```python
from build123d import *

# Parameters (mm, degrees)
SKETCH1_W           = 203.2
SKETCH1_H           = 60.2
BOSS_EXTRUDE1_DEPTH = 3
SKETCH5_R           = 2.5
CUT_EXTRUDE1_DEPTH  = 3
SKETCH7_R           = 2.5
CUT_EXTRUDE2_DEPTH  = 3
CUT_EXTRUDE3_DEPTH  = 3


with BuildPart() as part:
    # Sketch1 → Boss-Extrude1 (new body)
    with BuildSketch(Plane(origin=(0, 0, 0), x_dir=(1, 0, 0), z_dir=(0, 1, 0))):
        Rectangle(SKETCH1_W, SKETCH1_H)
    extrude(amount=BOSS_EXTRUDE1_DEPTH)

    # Sketch5 → Cut-Extrude1 (cut)
    with BuildSketch(Plane(origin=(0, 3, 0), x_dir=(1, 0, 0), z_dir=(0, 1, 0))):
        with Locations(Location((74.1, 3.6, 0), (0, 0, 270))):
            Circle(SKETCH5_R)
    extrude(amount=-CUT_EXTRUDE1_DEPTH, mode=Mode.SUBTRACT)

    # Sketch7 → Cut-Extrude2 (cut)
    with BuildSketch(Plane(origin=(0, 3, 0), x_dir=(1, 0, 0), z_dir=(0, 1, 0))):
        with Locations(Location((74.1, -7.1, 0), (0, 0, 270))):
            Circle(SKETCH7_R)
    extrude(amount=-CUT_EXTRUDE2_DEPTH, mode=Mode.SUBTRACT)

    # Sketch8 → Cut-Extrude3 (cut)
    with BuildSketch(Plane(origin=(0, 3, 0), x_dir=(1, 0, 0), z_dir=(0, 1, 0))):
        with BuildLine():
            Line((46.873111379, 15.864980996), (61.83445164, 0.932505799))
            ThreePointArc((61.83445164, 0.932505799), (61.836499957, -1.188813555), (59.715180603, -1.190861873))
            Line((59.715180603, -1.190861873), (44.753840342, 13.741613324))
            ThreePointArc((44.753840342, 13.741613324), (44.751792025, 15.862932678), (46.873111379, 15.864980996))
        make_face()
        with BuildLine():
            Line((36.873111379, 15.864980996), (51.83445164, 0.932505799))
            ThreePointArc((51.83445164, 0.932505799), (51.836499957, -1.188813555), (49.715180603, -1.190861873))
            Line((49.715180603, -1.190861873), (34.753840342, 13.741613324))
            ThreePointArc((34.753840342, 13.741613324), (34.751792025, 15.862932678), (36.873111379, 15.864980996))
        make_face()
        with BuildLine():
            Line((26.873111379, 15.864980996), (41.83445164, 0.932505799))
            ThreePointArc((41.83445164, 0.932505799), (41.836499957, -1.188813555), (39.715180603, -1.190861873))
            Line((39.715180603, -1.190861873), (24.753840342, 13.741613324))
            ThreePointArc((24.753840342, 13.741613324), (24.751792025, 15.862932678), (26.873111379, 15.864980996))
        make_face()
        with BuildLine():
            Line((16.873111379, 15.864980996), (31.83445164, 0.932505799))
            ThreePointArc((31.83445164, 0.932505799), (31.836499957, -1.188813555), (29.715180603, -1.190861873))
            Line((29.715180603, -1.190861873), (14.753840342, 13.741613324))
            ThreePointArc((14.753840342, 13.741613324), (14.751792025, 15.862932678), (16.873111379, 15.864980996))
        make_face()
        with BuildLine():
            Line((36.873111379, -4.135019004), (51.83445164, -19.067494201))
            ThreePointArc((51.83445164, -19.067494201), (51.836499957, -21.188813555), (49.715180603, -21.190861873))
            Line((49.715180603, -21.190861873), (34.753840342, -6.258386676))
            ThreePointArc((34.753840342, -6.258386676), (34.751792025, -4.137067322), (36.873111379, -4.135019004))
        make_face()
        with BuildLine():
            Line((26.873111379, -4.135019004), (41.83445164, -19.067494201))
            ThreePointArc((41.83445164, -19.067494201), (41.836499957, -21.188813555), (39.715180603, -21.190861873))
            Line((39.715180603, -21.190861873), (24.753840342, -6.258386676))
            ThreePointArc((24.753840342, -6.258386676), (24.751792025, -4.137067322), (26.873111379, -4.135019004))
        make_face()
        with BuildLine():
            Line((16.873111379, -4.135019004), (31.83445164, -19.067494201))
            ThreePointArc((31.83445164, -19.067494201), (31.836499957, -21.188813555), (29.715180603, -21.190861873))
            Line((29.715180603, -21.190861873), (14.753840342, -6.258386676))
            ThreePointArc((14.753840342, -6.258386676), (14.751792025, -4.137067322), (16.873111379, -4.135019004))
        make_face()
        with BuildLine():
            Line((46.873111379, -4.135019004), (61.83445164, -19.067494201))
            ThreePointArc((61.83445164, -19.067494201), (61.836499957, -21.188813555), (59.715180603, -21.190861873))
            Line((59.715180603, -21.190861873), (44.753840342, -6.258386676))
            ThreePointArc((44.753840342, -6.258386676), (44.751792025, -4.137067322), (46.873111379, -4.135019004))
        make_face()
    extrude(amount=-CUT_EXTRUDE3_DEPTH, mode=Mode.SUBTRACT)


solid = part.part
```
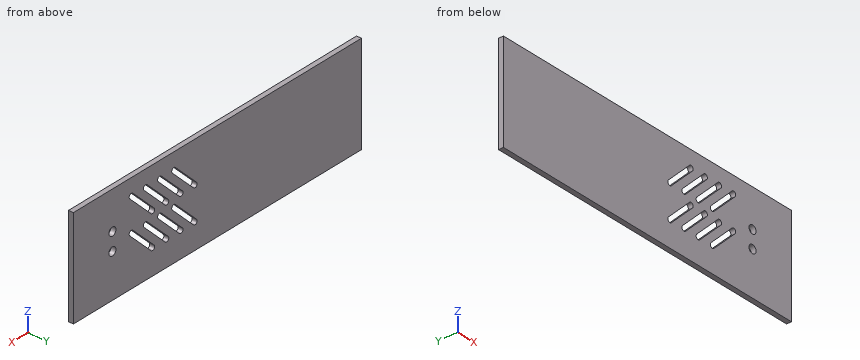
Geometry: final body of the model. Coordinates: model frame, mm. Round coordinates to 2 decimals unless told otherwise and drop trailing zeros. Order: outer loops, then holes, each group sorted by start corner. A loop starts at its lowest first (then second) coordinate and runs counter-clockwise, first axis right, second up. Notation, with made-up numbers: (25.5, 65.5) - (83.5, 65.5) arc R9 cw to (83.5, 69.5) - close; hole circle Ø7 at (34, -19). An arc over 180 degrees is marked (long way). Use CSV: the item, a comma, the result in double quotes. Start each with the question number.
Q1. Section query C-C (y = 0.65). State how many separate pieces and enclosed holes the cut face has, and give its area (3 significant figures).
Q2. Section query B-B (z = -3.6). Return loops of the section in (x, y).
Q3. First-contact query: pin 1 (6.5 mm diameter, centred on x = 74.1, z = 7.1, fed in from +Y). Flat tip, straight axial feed; report the tip coordinate or a pass-through.
Q4. Material intervals for line 1 along X through (y, z) = (1.8, 7.1); line 2 along X through (y, z) = (2.05, -12); line 3 along X through (y, z) = (2.7, 18.5), sorted ascending. Write a range as from..to.
Q5. Section query A-A (x = 74.1). Return loops of the section in (y, z).
Result set:
1,separate pieces,"1"
1,enclosed holes,"10"
1,area,"11,600 mm2"
2,outline,"(-101.6, 0) - (24.92, 0) - (24.92, 3) - (-101.6, 3) - close; (29.16, 0) - (34.92, 0) - (34.92, 3) - (29.16, 3) - close; (39.16, 0) - (44.92, 0) - (44.92, 3) - (39.16, 3) - close; (49.16, 0) - (54.92, 0) - (54.92, 3) - (49.16, 3) - close; (59.16, 0) - (71.6, 0) - (71.6, 3) - (59.16, 3) - close; (76.6, 0) - (101.6, 0) - (101.6, 3) - (76.6, 3) - close"
3,pin 1,"stops at y = 3"
4,line 1,"x = -101.6..15.6, 19.84..25.6, 29.84..35.6, 39.84..45.6, 49.84..71.6, 76.6..101.6"
4,line 2,"x = -101.6..16.5, 20.75..26.5, 30.75..36.5, 40.75..46.5, 50.75..101.6"
4,line 3,"x = -101.6..27.02, 31.27..37.02, 41.27..47.02, 51.27..57.02, 61.27..101.6"
5,outline,"(0, -30.1) - (3, -30.1) - (3, -6.1) - (0, -6.1) - close; (0, -1.1) - (3, -1.1) - (3, 4.6) - (0, 4.6) - close; (0, 9.6) - (3, 9.6) - (3, 30.1) - (0, 30.1) - close"
